Work out the finished part from the listing and answer in its coordinate system (mm). Coordinates: 2 decimals unless noted, no trailing zeros. Write each loop counter-clockwise with the first axis right and the second up, starting at its lowest first coordinate (ties: lowest second). Pieces come first, ordered by that corner, then holes. Notation, with made-up numbers: M -2.75,-18 L 3.25,-18 A33 ccw 3.25,21 Z; hole C -13.5,50 d2. An arc over 180 degrees is marked long. Use CSV: the item, a comma, the result in double quotes.
from build123d import *

# Parameters (mm, degrees)
F0_W        = 2.6332533453
F0_H        = 23.0305567384
F1_DEPTH    = 1.524
F2_SIZE     = 1
F3_SIZE     = 1
F4_T1_DEPTH = 13.8806275065
F5_T1_DEPTH = 12.7259269681
F6_SIZE     = 1
F7_T1_DEPTH = 98.6181021709
F8_SIZE     = 1
F9_T1_DEPTH = 98.6181021709


# Not quite as in the source:
# - a fillet or chamfer that OpenCascade refuses, or shapes differently, is made with other operations: its cross-section is extruded or revolved along the edge and cut away or added


with BuildPart() as f1:
    # F0 (on Front) → F1 (new body)
    with BuildSketch(Plane.XZ):
        Polygon((-4.1333585978, 47.5307323504), (4.1333585978, 47.5307323504), (4.3686307653, 47.5307323504), (0, 55.0974227954), (-4.3686307653, 47.5307323504), align=None)
        Polygon((4.1333585978, -47.5365004968), (4.1333585978, 47.5307323504), (-4.1333585978, 47.5307323504), (-4.1333585978, -47.5365004968), (-1.3166266726, -47.5365004968), (1.3166266726, -47.5365004968), align=None)
        with Locations((0, -59.051778866)):
            Rectangle(F0_W, F0_H)
    extrude(amount=F1_DEPTH)

    # F2
    f2_edges = [f1.edges().sort_by_distance(p)[0] for p in [
        (-2.184315, -1.524, 51.314078),
    ]]
    chamfer(f2_edges, length=F2_SIZE)

    # F3
    f3_edges = [f1.edges().sort_by_distance(p)[0] for p in [
        (2.472991, -1.524, 50.814078),
    ]]
    chamfer(f3_edges, length=F3_SIZE)

    # F4: chamfer of 1 on 1 edges, made by hand

    # F4_s2 → F4_t1 (cut)
    with BuildSketch(Plane(origin=(-18.2034116527, 0, 31.5292338535), x_dir=(0, 1, 0), z_dir=(-0.5, 0, 0.8660254038))):
        Polygon((-1, -27.5487113977), (0, -26.5487113977), (0, -27.5487113977), align=None)
    extrude(amount=F4_T1_DEPTH, mode=Mode.SUBTRACT)

    # F5: chamfer of 1 on 1 edges, made by hand

    # F5_s2 → F5_t1 (cut)
    with BuildSketch(Plane(origin=(24.5663751367, 0, 42.5502098946), x_dir=(0, 1, 0), z_dir=(-0.5, 0, -0.8660254038))):
        Polygon((0, -26.5487113977), (-1, -27.5487113977), (0, -27.5487113977), align=None)
    extrude(amount=F5_T1_DEPTH, mode=Mode.SUBTRACT)

    # F6
    f6_edges = [f1.edges().sort_by_distance(p)[0] for p in [
        (4.133359, -1.524, -0.799132),
    ]]
    chamfer(f6_edges, length=F6_SIZE)

    # F7: chamfer of 1 on 1 edges, made by hand

    # F7_s2 → F7_t1 (cut)
    with BuildSketch(Plane.XY.offset(-50.1081834848)):
        Polygon((4.1333585978, -1), (3.1333585978, 0), (4.1333585978, 0), align=None)
    extrude(amount=F7_T1_DEPTH, mode=Mode.SUBTRACT)

    # F8
    f8_edges = [f1.edges().sort_by_distance(p)[0] for p in [
        (-4.133359, 0, -0.799132),
    ]]
    chamfer(f8_edges, length=F8_SIZE)

    # F9: chamfer of 1 on 1 edges, made by hand

    # F9_s2 → F9_t1 (cut)
    with BuildSketch(Plane.XY.offset(-50.1081834848)):
        Polygon((-4.1333585978, -0.524), (-3.1333585978, -1.524), (-4.1333585978, -1.524), align=None)
    extrude(amount=F9_T1_DEPTH, mode=Mode.SUBTRACT)


solid = f1.part
Item 1: The part is cut by section B-B (y = -0.25). Write down the section's boundary in (x, z).
Answer:
outline,"M -3.38,-47.54 L -1.32,-47.54 L -1.32,-70.57 L 1.32,-70.57 L 1.32,-47.54 L 3.38,-47.54 L 3.38,47.74 L 0,53.6 L -3.38,47.74 Z"
Item 2: The part is cut by section A-A (z = 6.5). Write down the section's boundary in (x, y), then the cut area to 3 significant figures.
Answer:
outline,"M -3.9,-0.76 L -3.13,-1.52 L 3.13,-1.52 L 3.9,-0.76 L 3.13,0 L -3.13,0 Z"
area,"10.7 mm2"
Item 3: The part is cut by section C-C (z = -62). Write down the section's boundary in (x, y), then the cut area to 3 significant figures.
Answer:
outline,"M -1.32,-1.52 L 1.32,-1.52 L 1.32,0 L -1.32,0 Z"
area,"4.01 mm2"
Item 4: Consider probe 1 along Z at (x, y) = (3.25, -0.2); probe 2 along X at (y, z) = (-1.05, -57.5); probe 3 along X at (y, z) = (-0.65, -2.5). Determine where each line is inside the solid, lowest interval first.
Answer:
probe 1,"z = -47.54 to 47.87"
probe 2,"x = -1.32 to 1.32"
probe 3,"x = -3.78 to 3.78"
Item 5: Given pin 1 (0.8 mm diameter, centred on y = -1, z = -57.5, fed in from +X), flat-ended and moving along its own axis, determine where the tip first touches the part or whether it passes through.
Answer:
pin 1,"stops at x = 1.32"
